Part model, mm, in its own coordinate system. A direction names the side the tool comes from. Give positions to 0.01 mm unless a question says otherwise; leave off trailing zeros. Write each loop counter-clockwise with the first axis right and the second up, starting at its lowest first coordinate (ties: lowest second). Pieces come first, ordered by that corner, then holes. Notation, with made-up numbers: M -2.5,46 L 20.5,46 A23 ccw 20.5,62 Z; hole C -25,-1 d9. An arc over 180 degrees is marked long. Answer as CSV lines item,"result". Start each with the question number.
Item 1: Band-saw the part on B-B, the plane y = 23. List the corners of the cut face in (x, z), then the cut area to 3 significant figures.
Item 2: Wall check: L1, parallel to Y at x = -34, z = 22; L2, parallel to Y at x = -81.5, z = -22; L3, parallel to X at y = 37.5, z = 3. Give the ranges that are in metal, low to high. Write a range as from..to.
Item 3: 3-axis set-ups, long thin cutter, end or side, ignore diameter. For faces 1 (the cylindrical face through (-141.29, 6.06, 5.79)), 2 (the flat face through (-138.61, 12.76, -9.38)), 3 (the flat face through (-93.723, 93.54, 22.728)), 4 (the flat face through (-8, 49.784, -4)): which of +Z, -Z, +X, -X, +Y, -Y reach the whole face in a straight line?
Item 4: Pin check, flat tips, straight feed: pin 1 (3 mm diameter, centred on x = -89, z = -9.5, fed in from +Y); pin 2 (10 mm diameter, centred on y = 74.5, z = 2.5, fed in from -X); pin 3 (8 mm diameter, centred on y = 94, z = -5, fed in from -X). Stop position of each tip, or through.
Item 5: Two-plate mould, pull along X, no slides. Class faces 5 (the flat face through (-91, 59, -25.4)), 6 (the flat face through (-93.651, 89.285, 22.643)), 7 (the flat face through (-102.254, 91.435, 18.929)): +X half, -X half, draft (parallel to the pull), parting line (faces both ways), or undercut.
Item 6: Band-saw the part on C-C, the plane x = -140. Count the separate pieces of the cut face and the enclosed holes in it, then the cut area to 3 significant figures.
Item 7: Band-saw the part on A-A, the plane x = -3. List the corners of the cut face in (y, z).
from build123d import *

# Parameters (mm, degrees)
SKETCH1_W                              = 181.864
SKETCH1_H                              = 50.8
EXTRUDE1_DEPTH                         = 152.4
EXTRUDE2_DEPTH                         = 153.4
EXTRUDE3_DEPTH                         = 38.1
EXTRUDE4_DEPTH                         = 55.5498
SKETCH5_W                              = 54.61
SKETCH5_H                              = 50.8
EXTRUDE5_DEPTH                         = 7.9502
EXTRUDE6_DEPTH                         = 25.4
EXTRUDE7_DEPTH                         = 32.584173829
LPATTERN1_COUNT                        = 2
LPATTERN1_PITCH                        = 127
LPATTERN1_COUNT_DIR2                   = 2
LPATTERN1_PITCH_DIR2                   = 27.94
F_1_4_20_TAPPED_HOLE1_D                = 5.1054
F_1_4_20_TAPPED_HOLE1_DEPTH            = 16.51
F_1_4_20_TAPPED_HOLE1_CBORE_D          = 6.35
F_1_4_20_TAPPED_HOLE1_CBORE_DEPTH      = 12.7
F_1_4_20_TAPPED_HOLE1_TIP              = 1.533816902
EXTRUDE9_DEPTH                         = 128
CHAMFER1_SIZE                          = 2.54
CHAMFER2_SIZE                          = 15.24
EXTRUDE10_DEPTH                        = 32.584173829
SCREW_THRU_HOLE_AND_CBORE_D            = 15.4686
SCREW_THRU_HOLE_AND_CBORE_CBORE_D      = 35.56
SCREW_THRU_HOLE_AND_CBORE_CBORE_DEPTH  = 1.016
F_1_8_0_125_DIAMETER_HOLE1_D           = 3.19024
F_1_8_0_125_DIAMETER_HOLE1_DEPTH       = 9.525
F_1_8_0_125_DIAMETER_HOLE1_CSINK_D     = 5.334
F_1_8_0_125_DIAMETER_HOLE1_CSINK_ANGLE = 90
F_1_8_0_125_DIAMETER_HOLE1_TIP         = 0.958444791
CUT_EXTRUDE1_DEPTH                     = 9.525
CHAMFER3_SIZE                          = 1.0795
F_9_64_0_14063_DIAMETER_HOLE1_D        = 3.572002
F_9_64_0_14063_DIAMETER_HOLE1_DEPTH    = 43.18
F_1_16_0_0625_DIAMETER_HOLE1_D         = 1.5875
F_1_16_0_0625_DIAMETER_HOLE1_DEPTH     = 16.51


with BuildPart() as part:
    # Sketch1 → Extrude1 (new body)
    with BuildSketch(Plane(origin=(0, 0, 0), x_dir=(1, 0, 0), z_dir=(0, 1, 0))):
        with Locations((-65.532, 0)):
            Rectangle(SKETCH1_W, SKETCH1_H)
    extrude(amount=EXTRUDE1_DEPTH)

    # Sketch2 → Extrude2 (cut, through all)
    with BuildSketch(Plane(origin=(0, 152.4, 0), x_dir=(1, 0, 0), z_dir=(0, 1, 0))):
        Polygon((-156.464, -25.4), (-156.464, 25.4), (-147.50658938, 25.4), align=None)
    extrude(amount=-EXTRUDE2_DEPTH, mode=Mode.SUBTRACT)

    # Sketch3 → Extrude3 (cut)
    with BuildSketch(Plane(origin=(0, 152.4, 0), x_dir=(1, 0, 0), z_dir=(0, 1, 0))):
        Polygon((25.4, -25.4), (25.4, 25.4), (-124.39258938, 25.4), (-133.35, -25.4), align=None)
    extrude(amount=-EXTRUDE3_DEPTH, mode=Mode.SUBTRACT)

    # Sketch4 → Extrude4 (cut)
    with BuildSketch(Plane(origin=(0, 114.3, 0), x_dir=(1, 0, 0), z_dir=(0, 1, 0))):
        Polygon((25.4, -25.4), (-95.25, -25.4), (-58.42, 18.492284815), (-58.42, 25.4), (25.4, 25.4), align=None)
    extrude(amount=-EXTRUDE4_DEPTH, mode=Mode.SUBTRACT)

    # Sketch5 → Extrude5 (cut)
    with BuildSketch(Plane(origin=(0, 58.7502, 0), x_dir=(1, 0, 0), z_dir=(0, 1, 0))):
        with Locations((-1.905, 0)):
            Rectangle(SKETCH5_W, SKETCH5_H)
    extrude(amount=-EXTRUDE5_DEPTH, mode=Mode.SUBTRACT)

    # Sketch6 → Extrude6 (cut)
    with BuildSketch(Plane.XZ):
        Polygon((25.4, 25.4), (25.4, -25.4), (-124.39258938, -25.4), (-133.35, 25.4), align=None)
    extrude(amount=-EXTRUDE6_DEPTH, mode=Mode.SUBTRACT)

    # Sketch7 → Extrude7 (cut, through all)
    with BuildSketch(Plane(origin=(-124.985349671, 0, -22.03828934), x_dir=(0.173648178, 0, -0.984807753), z_dir=(0.984807753, 0, 0.173648178))):
        with BuildLine():
            Line((-35.635705397, 142.9766), (-35.635705397, 136.6266))
            ThreePointArc((-35.635705397, 136.6266), (-39.204405397, 133.0579), (-42.773105397, 136.6266))
            Line((-42.773105397, 136.6266), (-42.773105397, 142.9766))
            ThreePointArc((-42.773105397, 142.9766), (-39.204405397, 146.5453), (-35.635705397, 142.9766))
        make_face()
    extrude7 = extrude(amount=-EXTRUDE7_DEPTH, mode=Mode.SUBTRACT)

    # LPattern1: Extrude7 2 × 2, 1 skipped
    with Locations(*[Vector(0, -1, 0) * (i * LPATTERN1_PITCH) + Vector(0.173648178, 0, -0.984807753) * (j * LPATTERN1_PITCH_DIR2) for i in range(LPATTERN1_COUNT) for j in range(LPATTERN1_COUNT_DIR2) if (i, j) not in ((0, 0), (1, 0))]):
        add(extrude7, mode=Mode.SUBTRACT)

    # 1/4-20 Tapped Hole1
    with Locations(Plane(origin=(-43.387935998, 0, -36.406801094), x_dir=(0.64278761, 0, -0.766044443), z_dir=(0.766044443, 0, 0.64278761))):
        with Locations((-49.822048678, 104.648), (-49.822048678, 71.628)):
            CounterBoreHole(F_1_4_20_TAPPED_HOLE1_D / 2, F_1_4_20_TAPPED_HOLE1_CBORE_D / 2, F_1_4_20_TAPPED_HOLE1_CBORE_DEPTH, depth=F_1_4_20_TAPPED_HOLE1_DEPTH)
            with Locations((0, 0, -(F_1_4_20_TAPPED_HOLE1_DEPTH + F_1_4_20_TAPPED_HOLE1_TIP / 2))):  # 118° drill point
                Cone(0, F_1_4_20_TAPPED_HOLE1_D / 2, F_1_4_20_TAPPED_HOLE1_TIP, mode=Mode.SUBTRACT)

    # Sketch19 → Extrude9 (cut, through all)
    with BuildSketch(Plane.XZ.offset(-25.4)):
        with BuildLine():
            Line((27.94, 25.4), (0, 25.4))
            ThreePointArc((0, 25.4), (25.4, 0), (0, -25.4))
            Line((0, -25.4), (27.94, -25.4))
            Line((27.94, -25.4), (27.94, 25.4))
        make_face()
    extrude(amount=-EXTRUDE9_DEPTH, mode=Mode.SUBTRACT)

    # Chamfer1
    chamfer1_edges = [part.edges().sort_by_distance(p)[0] for p in [
        (-135.94958938, 152.4, -25.4),
        (-144.907, 0, 25.4),
        (-29.21, 54.7751, 25.4),
        (-29.21, 54.7751, -25.4),
        (-135.94958938, 0, -25.4),
        (-144.907, 152.4, 25.4),
    ]]
    chamfer(chamfer1_edges, length=CHAMFER1_SIZE)

    # Chamfer2
    chamfer2_edges = [part.edges().sort_by_distance(p)[0] for p in [
        (-58.42, 114.3, -21.946142408),
    ]]
    chamfer(chamfer2_edges, length=CHAMFER2_SIZE)

    # Sketch20 → Extrude10 (cut, through all)
    with BuildSketch(Plane(origin=(-124.985349671, 0, -22.03828934), x_dir=(0.173648178, 0, -0.984807753), z_dir=(0.984807753, 0, 0.173648178))):
        with BuildLine():
            Line((-26.745705397, 15.9766), (-26.745705397, 9.6266))
            ThreePointArc((-26.745705397, 9.6266), (-30.314405397, 6.0579), (-33.883105397, 9.6266))
            Line((-33.883105397, 9.6266), (-33.883105397, 15.9766))
            ThreePointArc((-33.883105397, 15.9766), (-30.314405397, 19.5453), (-26.745705397, 15.9766))
        make_face()
    extrude(amount=-EXTRUDE10_DEPTH, mode=Mode.SUBTRACT)

    # SCREW THRU HOLE AND CBORE (through all)
    with Locations(Plane(origin=(0, 50.8, 0), x_dir=(-1, 0, 0), z_dir=(0, 1, 0))):
        with Locations((0, 0)):
            CounterBoreHole(SCREW_THRU_HOLE_AND_CBORE_D / 2, SCREW_THRU_HOLE_AND_CBORE_CBORE_D / 2, SCREW_THRU_HOLE_AND_CBORE_CBORE_DEPTH)

    # 1/8 (0.125) Diameter Hole1
    with Locations(Plane(origin=(-43.387935998, 0, -36.406801094), x_dir=(0.64278761, 0, -0.766044443), z_dir=(0.766044443, 0, 0.64278761))):
        with Locations((-49.784, 91.412613047)):
            CounterSinkHole(F_1_8_0_125_DIAMETER_HOLE1_D / 2, F_1_8_0_125_DIAMETER_HOLE1_CSINK_D / 2, depth=F_1_8_0_125_DIAMETER_HOLE1_DEPTH, counter_sink_angle=F_1_8_0_125_DIAMETER_HOLE1_CSINK_ANGLE)
            with Locations((0, 0, -(F_1_8_0_125_DIAMETER_HOLE1_DEPTH + F_1_8_0_125_DIAMETER_HOLE1_TIP / 2))):  # 118° drill point
                Cone(0, F_1_8_0_125_DIAMETER_HOLE1_D / 2, F_1_8_0_125_DIAMETER_HOLE1_TIP, mode=Mode.SUBTRACT)

    # Sketch26 → Cut-Extrude1 (cut)
    with BuildSketch(Plane(origin=(-43.387935998, 0, -36.406801094), x_dir=(0.64278761, 0, -0.766044443), z_dir=(0.766044443, 0, 0.64278761))):
        with BuildLine():
            Line((-73.6092, 89.817493047), (-92.6592, 89.817493047))
            ThreePointArc((-92.6592, 89.817493047), (-94.25432, 91.412613047), (-92.6592, 93.007733047))
            Line((-92.6592, 93.007733047), (-73.6092, 93.007733047))
            ThreePointArc((-73.6092, 93.007733047), (-72.01408, 91.412613047), (-73.6092, 89.817493047))
        make_face()
    extrude(amount=-CUT_EXTRUDE1_DEPTH, mode=Mode.SUBTRACT)

    # Chamfer3
    chamfer3_edges = [part.edges().sort_by_distance(p)[0] for p in [
        (-92.976508859, 89.817493047, 22.690558764),
        (-92.976508859, 93.007733047, 22.690558764),
        (-89.677694345, 91.412613047, 18.759184717),
    ]]
    chamfer(chamfer3_edges, length=CHAMFER3_SIZE)

    # 9/64 (0.14063) Diameter Hole1
    with Locations(Plane(origin=(0, 114.3, 0), x_dir=(-1, 0, 0), z_dir=(0, 1, 0))):
        with Locations((89.235297248, -9.839239495)):
            Hole(F_9_64_0_14063_DIAMETER_HOLE1_D / 2, depth=F_9_64_0_14063_DIAMETER_HOLE1_DEPTH)

    # 1/16 (0.0625) Diameter Hole1
    with Locations(Plane(origin=(-43.387935998, 0, -36.406801094), x_dir=(0.64278761, 0, -0.766044443), z_dir=(0.766044443, 0, 0.64278761))):
        with Locations((-49.784, 91.412613047)):
            Hole(F_1_16_0_0625_DIAMETER_HOLE1_D / 2, depth=F_1_16_0_0625_DIAMETER_HOLE1_DEPTH)


solid = part.part
Output:
1,outline,"M -156.46,25.4 L -147.51,-25.4 L -124.39,-25.4 L -133.35,25.4 Z"
1,area,"1,170 mm²"
2,L1,"25.4..58.75"
2,L2,"25.4..114.3"
2,L3,"-152.51..-7.13, 7.13..25.22"
3,face 1,"none"
3,face 2,"+X"
3,face 3,"+Z, +X"
3,face 4,"+Y"
4,pin 1,"y = 114.3"
4,pin 2,"x = -153.31"
4,pin 3,"x = -151.81"
5,face 5,"draft"
5,face 6,"+X half"
5,face 7,"undercut"
6,separate pieces,"1"
6,enclosed holes,"4"
6,area,"7,380 mm²"
7,outline,"M 25.4,-25.4 L 50.8,-25.4 L 50.8,-17.53 L 49.78,-17.53 L 49.78,-7.13 L 25.4,-7.13 Z; M 25.4,7.13 L 49.78,7.13 L 49.78,17.53 L 50.8,17.53 L 50.8,25.4 L 25.4,25.4 Z"
